```python
from build123d import *

# Parameters (mm, degrees)
SKETCH1_W                                            = 207
SKETCH1_H                                            = 122.7
SKETCH1_W_2                                          = 167
SKETCH1_H_2                                          = 102.7
EXTRUDE1_DEPTH                                       = 12
FILLET1_R                                            = 10
CHAMFER1_SIZE                                        = 1
SKETCH2_W                                            = 186.9
SKETCH2_H                                            = 106
EXTRUDE2_DEPTH                                       = 2
FILLET2_R                                            = 2.5
SKETCH3_W                                            = 195
SKETCH3_H                                            = 112.7
EXTRUDE3_DEPTH                                       = 3.5
F_2_0_2_DIAMETER_HOLE1_D                             = 2
CSK_FOR_M3_COUNTERSUNK_RAISED_HEAD_SCREW_D           = 3.4
CSK_FOR_M3_COUNTERSUNK_RAISED_HEAD_SCREW_CSINK_D     = 6.3
CSK_FOR_M3_COUNTERSUNK_RAISED_HEAD_SCREW_CSINK_ANGLE = 90
CHAMFER2_SIZE                                        = 2
SKETCH12_W                                           = 30
SKETCH12_H                                           = 2
EXTRUDE4_DEPTH                                       = 1.5
FILLET3_R                                            = 1
SKETCH13_W                                           = 30
SKETCH13_H                                           = 2
EXTRUDE5_DEPTH                                       = 1.5
FILLET4_R                                            = 1
SKETCH14_W                                           = 30
SKETCH14_H                                           = 2
EXTRUDE6_DEPTH                                       = 1.5
FILLET5_R                                            = 1
SKETCH15_W                                           = 30
SKETCH15_H                                           = 2
EXTRUDE7_DEPTH                                       = 1.5
FILLET6_R                                            = 1


with BuildPart() as part:
    # Sketch1 → Extrude1 (new body)
    with BuildSketch(Plane(origin=(0, 0, 0), x_dir=(1, 0, 0), z_dir=(0, 1, 0))):
        Rectangle(SKETCH1_W, SKETCH1_H)
        Rectangle(SKETCH1_W_2, SKETCH1_H_2, mode=Mode.SUBTRACT)
    extrude(amount=EXTRUDE1_DEPTH)

    # Fillet1
    fillet1_edges = [part.edges().sort_by_distance(p)[0] for p in [
        (-103.5, 6, -61.35),
        (103.5, 6, -61.35),
        (103.5, 6, 61.35),
        (-103.5, 6, 61.35),
    ]]
    fillet(fillet1_edges, radius=FILLET1_R)

    # Chamfer1
    chamfer1_edges = [part.edges().sort_by_distance(p)[0] for p in [
        (-83.5, 12, 0),
        (0, 12, 51.35),
        (83.5, 12, 0),
        (0, 12, -51.35),
        (103.5, 12, 0),
        (0, 12, 61.35),
        (-103.5, 12, 0),
        (0, 12, -61.35),
        (-100.571067812, 12, 58.421067812),
        (-100.571067812, 12, -58.421067812),
        (100.571067812, 12, -58.421067812),
        (100.571067812, 12, 58.421067812),
    ]]
    chamfer(chamfer1_edges, length=CHAMFER1_SIZE)

    # Sketch2 → Extrude2 (cut)
    with BuildSketch(Plane.XZ):
        Rectangle(SKETCH2_W, SKETCH2_H)
    extrude(amount=-EXTRUDE2_DEPTH, mode=Mode.SUBTRACT)

    # Fillet2
    fillet2_edges = [part.edges().sort_by_distance(p)[0] for p in [
        (-93.45, 1, -53),
        (-93.45, 1, 53),
        (93.45, 1, 53),
        (93.45, 1, -53),
    ]]
    fillet(fillet2_edges, radius=FILLET2_R)

    # Sketch3 → Extrude3 (add)
    with BuildSketch(Plane.XZ):
        Rectangle(SKETCH3_W, SKETCH3_H)
        with BuildLine():
            Line((-90.95, -53), (90.95, -53))
            ThreePointArc((90.95, -53), (92.717766953, -52.267766953), (93.45, -50.5))
            Line((93.45, -50.5), (93.45, 50.5))
            ThreePointArc((93.45, 50.5), (92.717766953, 52.267766953), (90.95, 53))
            Line((90.95, 53), (-90.95, 53))
            ThreePointArc((-90.95, 53), (-92.717766953, 52.267766953), (-93.45, 50.5))
            Line((-93.45, 50.5), (-93.45, -50.5))
            ThreePointArc((-93.45, -50.5), (-92.717766953, -52.267766953), (-90.95, -53))
        make_face(mode=Mode.SUBTRACT)
    extrude(amount=EXTRUDE3_DEPTH)

    # Ø2.0 (2) Diameter Hole1 (through all)
    with Locations(Plane(origin=(-103.5, 2, 61.35), x_dir=(1, 0, 0), z_dir=(0, -1, 0))):
        with Locations((190.95, -14.05), (190.95, -108.05), (16.05, -108.05), (16.05, -14.05)):
            Hole(F_2_0_2_DIAMETER_HOLE1_D / 2)

    # CSK for M3 Countersunk Raised Head Screw2 (through all)
    with Locations(Plane(origin=(0, 12, 0), x_dir=(1, 0, 0), z_dir=(0, 1, 0))):
        with Locations((87.45, 46.7), (87.45, -47.3), (-87.45, -47.3), (-87.45, 46.7)):
            CounterSinkHole(CSK_FOR_M3_COUNTERSUNK_RAISED_HEAD_SCREW_D / 2, CSK_FOR_M3_COUNTERSUNK_RAISED_HEAD_SCREW_CSINK_D / 2, counter_sink_angle=CSK_FOR_M3_COUNTERSUNK_RAISED_HEAD_SCREW_CSINK_ANGLE)

    # Chamfer2
    chamfer2_edges = [part.edges().sort_by_distance(p)[0] for p in [
        (-97.5, -1.75, 56.35),
        (-97.5, -1.75, -56.35),
        (97.5, -1.75, -56.35),
        (97.5, -1.75, 56.35),
    ]]
    chamfer(chamfer2_edges, length=CHAMFER2_SIZE)

    # Sketch12 → Extrude4 (add)
    with BuildSketch(Plane.ZY.offset(97.5)):
        with Locations((0, -2.5)):
            Rectangle(SKETCH12_W, SKETCH12_H)
    extrude(amount=EXTRUDE4_DEPTH)

    # Fillet3
    fillet3_edges = [part.edges().sort_by_distance(p)[0] for p in [
        (-99, -3.5, 0),
        (-99, -1.5, 0),
    ]]
    fillet(fillet3_edges, radius=FILLET3_R - 0.0001)  # a hair under: the kernel refuses the full size

    # Sketch13 → Extrude5 (add)
    with BuildSketch(Plane(origin=(97.5, 0, 0), x_dir=(0, 0, -1), z_dir=(1, 0, 0))):
        with Locations((0, -2.5)):
            Rectangle(SKETCH13_W, SKETCH13_H)
    extrude(amount=EXTRUDE5_DEPTH)

    # Fillet4
    fillet4_edges = [part.edges().sort_by_distance(p)[0] for p in [
        (99, -1.5, 0),
        (99, -3.5, 0),
    ]]
    fillet(fillet4_edges, radius=FILLET4_R - 0.0001)  # a hair under: the kernel refuses the full size

    # Sketch14 → Extrude6 (add)
    with BuildSketch(Plane.XY.offset(56.35)):
        with Locations((0, -2.5)):
            Rectangle(SKETCH14_W, SKETCH14_H)
    extrude(amount=EXTRUDE6_DEPTH)

    # Fillet5
    fillet5_edges = [part.edges().sort_by_distance(p)[0] for p in [
        (0, -3.5, 57.85),
        (0, -1.5, 57.85),
    ]]
    fillet(fillet5_edges, radius=FILLET5_R - 0.0001)  # a hair under: the kernel refuses the full size

    # Sketch15 → Extrude7 (add)
    with BuildSketch(Plane(origin=(0, 0, -56.35), x_dir=(-1, 0, 0), z_dir=(0, 0, -1))):
        with Locations((0, -2.5)):
            Rectangle(SKETCH15_W, SKETCH15_H)
    extrude(amount=EXTRUDE7_DEPTH)

    # Fillet6
    fillet6_edges = [part.edges().sort_by_distance(p)[0] for p in [
        (0, -3.5, -57.85),
        (0, -1.5, -57.85),
    ]]
    fillet(fillet6_edges, radius=FILLET6_R - 0.0001)  # a hair under: the kernel refuses the full size


solid = part.part
```
Read the model definition and answer for the solid it produces. Units are mm, in the model's axes. A direction names the side the tool comes from. Give positions to 0.01 mm unless a question says otherwise; leave off trailing zeros. Write each loop counter-clockwise with the first axis right and the second up, starting at its lowest first coordinate (ties: lowest second). Pieces come first, ordered by that corner, then holes. Notation, with made-up numbers: M 63.5,69 L 116.5,69 A16 cw 116.5,94 Z; hole C 37.25,68.5 d4. An arc over 180 degrees is marked long. Put each result on its own line as item: value. Start each with the question number.
1. Which of the six approach directions +Z, -Z, +X, -X, +Y, -Y give full straight-line access (tool end or side, diameter ignored) to faces 1 (the flat face through (-84, 2, 0)), 2 (the conical face through (99.915, 11.826, 57.908)), 3 (the flat face through (-83.5, 6, 1))?
2. For a pull along X with two mould halves and no side action, classify faces 4 (the conical face through (-99.915, 11.826, -57.908)), 5 (the flat face through (1, -1, 53)), 6 (the flat face through (-1, 5, 61.35)) as released by +X, released by -X, zero draft, split by the parting line, or undercut.
3. The part is cut by section D-D, the plane x = -64.5. Give the vertices of the cut face in (y, z).
4. The part is cut by section C-C, the plane z = -37.5. Give the vertices of the cut face in (x, y), and give its area (3 significant figures).
5. Each of these flat-tipped pins is pushed along its axis until it touches: pin 1 Ø6 at (x, y) = (-73.5, -1) entering from +Z; pin 2 Ø1.6 at (y, z) = (-2.5, 57.5) entering from +X; pin 3 Ø1.8 at (y, z) = (-1, -27) entering from -X; pin 4 Ø1.2 at (y, z) = (-2.5, -57) entering from -X. Where does it stop, or does it pass through?
6. Consider line 1 along X through (y, z) = (8, 47.3); line 2 along Z through (x, y) = (-87.45, 4.25); line 3 along X through (y, z) = (2.75, 17). Determine where each line is inside the solid, lowest interval first.
Final values:
1. face 1: -Y
1. face 2: +Z, +X, +Y
1. face 3: +Y, -Y
2. face 4: released by -X
2. face 5: undercut
2. face 6: zero draft
3. outline: M -3.5,-56.35 L 0,-56.35 L 0,-61.35 L 11,-61.35 L 12,-60.35 L 12,-52.35 L 11,-51.35 L 2,-51.35 L 2,-53 L -3.5,-53 Z; M -3.5,53 L 2,53 L 2,51.35 L 11,51.35 L 12,52.35 L 12,60.35 L 11,61.35 L 0,61.35 L 0,56.35 L -3.5,56.35 Z
4. outline: M -103.5,0 L -97.5,0 L -97.5,-3.5 L -93.45,-3.5 L -93.45,2 L -83.5,2 L -83.5,11 L -84.5,12 L -102.5,12 L -103.5,11 Z; M 83.5,2 L 93.45,2 L 93.45,-3.5 L 97.5,-3.5 L 97.5,0 L 103.5,0 L 103.5,11 L 102.5,12 L 84.5,12 L 83.5,11 Z
4. area: 467 mm²
5. pin 1: stops at z = 61.35
5. pin 2: stops at x = 15
5. pin 3: stops at x = -97.5
5. pin 4: stops at x = -15
6. line 1: x = -103.5 to -89.15, -85.75 to -83.5, 83.5 to 85.75, 89.15 to 103.5
6. line 2: z = -61.35 to -48.4, -45 to 45.6, 49 to 61.35
6. line 3: x = -103.5 to -83.5, 83.5 to 103.5
